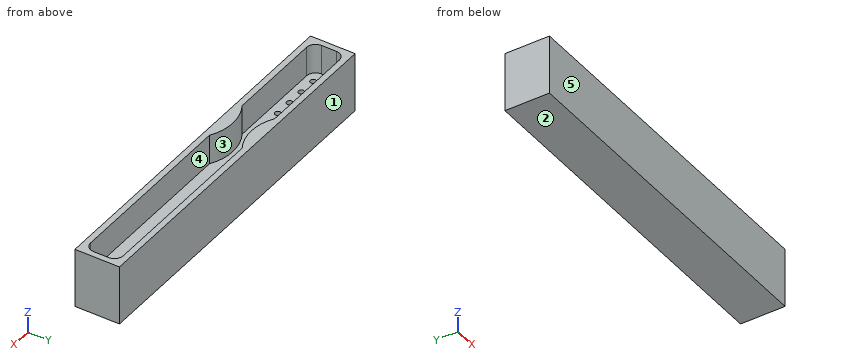
from build123d import *

# Parameters (mm, degrees)
F0_W     = 120
F0_H     = 15
F1_DEPTH = 20
F3_DEPTH = 10
F4_R     = 1
F5_DEPTH = 5


with BuildPart() as f1:
    # F0 (on Top) → F1 (new body)
    with BuildSketch(Plane.XY):
        with Locations((47.004177, -6.222026)):
            Rectangle(F0_W, F0_H)
    extrude(amount=F1_DEPTH)

    # F2 (on face) → F3 (cut)
    with BuildSketch(Plane.XY.offset(20)):
        with BuildLine():
            Line((24.868954, -0.722026), (-7.995823, -0.722026))
            ThreePointArc((-7.995823, -0.722026), (-10.117143, -1.600706), (-10.995823, -3.722026))
            Line((-10.995823, -3.722026), (-10.995823, -6.222026))
            Line((-10.995823, -6.222026), (105.004177, -6.222026))
            Line((105.004177, -6.222026), (105.004177, -3.722026))
            ThreePointArc((105.004177, -3.722026), (104.125498, -1.600706), (102.004177, -0.722026))
            Line((102.004177, -0.722026), (41.503951, -0.722026))
            ThreePointArc((41.503951, -0.722026), (33.186452, -3.06816), (24.868954, -0.722026))
        make_face()
        with BuildLine():
            Line((105.004177, -6.222026), (-10.995823, -6.222026))
            Line((-10.995823, -6.222026), (-10.995823, -8.722026))
            ThreePointArc((-10.995823, -8.722026), (-10.117143, -10.843347), (-7.995823, -11.722026))
            Line((-7.995823, -11.722026), (24.868954, -11.722026))
            ThreePointArc((24.868954, -11.722026), (33.186452, -9.375893), (41.503951, -11.722026))
            Line((41.503951, -11.722026), (102.004177, -11.722026))
            ThreePointArc((102.004177, -11.722026), (104.125498, -10.843347), (105.004177, -8.722026))
            Line((105.004177, -8.722026), (105.004177, -6.222026))
        make_face()
    extrude(amount=-F3_DEPTH, mode=Mode.SUBTRACT)

    # F4 (on face) → F5 (cut)
    with BuildSketch(Plane.XY.offset(10)):
        with Locations((-6.801731, -3.722026)):
            Circle(F4_R)
        with Locations((-0.801731, -3.722026)):
            Circle(F4_R)
        with Locations((5.198269, -3.722026)):
            Circle(F4_R)
        with Locations((11.198269, -3.722026)):
            Circle(F4_R)
        with Locations((11.198269, -8.722026)):
            Circle(F4_R)
        with Locations((5.198269, -8.722026)):
            Circle(F4_R)
        with Locations((-0.801731, -8.722026)):
            Circle(F4_R)
        with Locations((-6.801731, -8.722026)):
            Circle(F4_R)
    extrude(amount=-F5_DEPTH, mode=Mode.SUBTRACT)


solid = f1.part
Design review of the part built by this model. Coordinates are the model's own, in mm. Face numbers are marked on the shaded views. A direction names the side the tool comes from. Give positions to 0.01 mm unless a question says otherwise; leave off trailing zeros. Loops run counter-clockwise (first coordinate to the right, second up) from the corner with the lowest first, then second, coordinate; pieces in that order, holes last. Notation, with made-up numbers: (56.25, -2.5) - (94.25, -2.5) arc R13 ccw to (94.25, 4.5) - close; hole circle Ø9 at (-35, 29.25). An arc over 180 degrees is marked (long way). Write item = value, one per line.
1) Clearance check with flat-ended pins moving along their axes: pin 1 Ø8 at (x, y) = (75, -7.5) entering from +Z; pin 2 Ø2.5 at (x, y) = (11.2, -8.72) entering from -Z; pin 3 Ø1.2 at (x, y) = (-0.8, -3.72) entering from +Z. State where each tip first meets the part, or that it passes through.
Result sheet:
pin_1 = 10
pin_2 = 0
pin_3 = 5
2) Take a section at C-C on x = 39. State the section outline as (y, z) points, and give its area (3 significant figures).
Result sheet:
outline = (-13.72, 0) - (1.28, 0) - (1.28, 20) - (-1.97, 20) - (-1.97, 10) - (-10.48, 10) - (-10.48, 20) - (-13.72, 20) - close
area = 215 mm2
3) To check wall thickness, follow line 1 (Y direction, x = 5, z = 13.25); line 2 (X direction, y = -4.5, z = 12.5); line 3 (X direction, y = -1.25, z = 17.25). State the ranges of each line that lie inside material, in increasing order.
Result sheet:
line_1 = -13.72 to -11.72, -0.72 to 1.28
line_2 = -13 to -11, 105 to 107
line_3 = -13 to -9.7, 25.8 to 40.57, 103.7 to 107
4) Tool access review of the marked faces 4 and 5: name each direction out of +Z, -Z, +X, -X, +Y, -Y from which nothing blocks a thin tool from reaching the whole face with its end or side.
Result sheet:
face_4 = +Z
face_5 = +Z, -Z, +X, -X, -Y
5) Draft analysis for pull direction Y (two halves, no side actions). For the marked faces 1, 2 and 3, state which applies: +Y half, -Y half, draft (parallel to the pull), parting line (faces both ways), or undercut.
Result sheet:
face_1 = +Y half
face_2 = draft
face_3 = undercut
6) Take a section at A-A on z = 14. State the section outline as (x, y) points, and give its area (3 significant figures).
Result sheet:
outline = (-13, -13.72) - (107, -13.72) - (107, 1.28) - (-13, 1.28) - close; hole (-11, -8.72) arc R3 ccw to (-8, -11.72) - (24.87, -11.72) arc R15.92 cw to (41.5, -11.72) - (102, -11.72) arc R3 ccw to (105, -8.72) - (105, -3.72) arc R3 ccw to (102, -0.72) - (41.5, -0.72) arc R15.92 cw to (24.87, -0.72) - (-8, -0.72) arc R3 ccw to (-11, -3.72) - close
area = 585 mm2
7) Take a section at B-B on x = 21.5. State the section outline as (y, z) points, and give its area (3 significant figures).
Result sheet:
outline = (-13.72, 0) - (1.28, 0) - (1.28, 20) - (-0.72, 20) - (-0.72, 10) - (-11.72, 10) - (-11.72, 20) - (-13.72, 20) - close
area = 190 mm2
